from build123d import *

# Parameters (mm, degrees)
SKETCH2_R           = 15
SKETCH1_R           = 25
SKETCH3_R           = 15
BOSS_EXTRUDE1_DEPTH = 5
FILLET1_R           = 10
SKETCH4_R           = 1.75
CUT_EXTRUDE1_DEPTH  = 130
SKETCH5_R           = 4
CUT_EXTRUDE2_DEPTH  = 130
SKETCH6_R           = 22
BOSS_EXTRUDE2_DEPTH = 4
SKETCH7_R           = 17
BOSS_EXTRUDE3_DEPTH = 20
SKETCH15_W          = 8.431609766
SKETCH15_H          = 4
SKETCH15_W_2        = 8.578672696
SKETCH18_R          = 12.5
CUT_EXTRUDE5_DEPTH  = 20
SKETCH19_R          = 47.987160243
CUT_EXTRUDE6_DEPTH  = 44.301270362
SKETCH20_R          = 1.75
BOSS_EXTRUDE5_DEPTH = 4
CIRPATTERN3_COUNT   = 4
FILLET2_R           = 10
CHAMFER1_SIZE       = 0.5
SKETCH22_W          = 15
SKETCH22_H          = 8
BOSS_EXTRUDE6_DEPTH = 7.5
CHAMFER2_SIZE       = 3
CHAMFER3_SIZE       = 0.5
CUT_EXTRUDE8_START  = -0.1
SKETCH24_R          = 41.017326151
SKETCH24_R_2        = 17
CUT_EXTRUDE8_DEPTH  = 0.1
CHAMFER4_SIZE       = 0.5


with BuildPart() as part:
    # Sketch2 → Loft1 section 0
    with BuildSketch(Plane.XY.offset(20)):
        Circle(SKETCH2_R)
    # Sketch1 → Loft1 section 1
    with BuildSketch(Plane.XY):
        Circle(SKETCH1_R)
    loft()

    # Sketch3 → Boss-Extrude1 (add)
    with BuildSketch(Plane.XY.offset(20)):
        Circle(SKETCH3_R)
    extrude(amount=BOSS_EXTRUDE1_DEPTH)

    # Fillet1
    fillet1_edges = [part.edges().sort_by_distance(p)[0] for p in [
        (-15, 0, 20),
    ]]
    fillet(fillet1_edges, radius=FILLET1_R)

    # Sketch4 → Cut-Extrude1 (cut)
    with BuildSketch(Plane(origin=(0, 0, 0), x_dir=(-1, 0, 0), z_dir=(0, 0, -1))):
        with Locations((0, 20)):
            Circle(SKETCH4_R)
        with Locations((-20, 0)):
            Circle(SKETCH4_R)
        with Locations((0, -20)):
            Circle(SKETCH4_R)
        with Locations((20, 0)):
            Circle(SKETCH4_R)
    extrude(amount=-CUT_EXTRUDE1_DEPTH, mode=Mode.SUBTRACT)

    # Sketch5 → Cut-Extrude2 (cut)
    with BuildSketch(Plane(origin=(0, 0, 3), x_dir=(-1, 0, 0), z_dir=(0, 0, -1))):
        with Locations((0, 20)):
            Circle(SKETCH5_R)
        with Locations((20, 0)):
            Circle(SKETCH5_R)
        with Locations((-20, 0)):
            Circle(SKETCH5_R)
        with Locations((0, -20)):
            Circle(SKETCH5_R)
    extrude(amount=-CUT_EXTRUDE2_DEPTH, mode=Mode.SUBTRACT)

    # Sketch6 → Boss-Extrude2 (add)
    with BuildSketch(Plane.XY.offset(25)):
        Circle(SKETCH6_R)
    extrude(amount=BOSS_EXTRUDE2_DEPTH)

    # Sketch7 → Boss-Extrude3 (add)
    with BuildSketch(Plane.XY.offset(29)):
        Circle(SKETCH7_R)
    extrude(amount=BOSS_EXTRUDE3_DEPTH)

    # Sketch15 → Cut-Revolve1 (revolve, cut)
    with BuildSketch(Plane(origin=(0, 0, 0), x_dir=(1, 0, 0), z_dir=(0, 1, 0))):
        with Locations((-17.215804883, -35)):
            Rectangle(SKETCH15_W, SKETCH15_H)
        with Locations((-17.289336348, -43)):
            Rectangle(SKETCH15_W_2, SKETCH15_H)
    revolve(axis=Axis((0, 0, 29), (0, 0, 1)), mode=Mode.SUBTRACT)

    # Sketch18 → Cut-Extrude5 (cut)
    with BuildSketch(Plane(origin=(0, 0, 0), x_dir=(-1, 0, 0), z_dir=(0, 0, -1))):
        Circle(SKETCH18_R)
    extrude(amount=-CUT_EXTRUDE5_DEPTH, mode=Mode.SUBTRACT)

    # Sketch19 → Cut-Extrude6 (cut, through all)
    with BuildSketch(Plane(origin=(0, 0, 25), x_dir=(-1, 0, 0), z_dir=(0, 0, -1))):
        Circle(SKETCH19_R)
    extrude(amount=CUT_EXTRUDE6_DEPTH, mode=Mode.SUBTRACT)

    # Sketch20 → Boss-Extrude5 (add)
    with BuildSketch(Plane(origin=(0, 0, 25), x_dir=(-1, 0, 0), z_dir=(0, 0, -1))):
        with BuildLine():
            Line((-4, 30), (-4, 21.633307653))
            ThreePointArc((-4, 21.633307653), (0, 22), (4, 21.633307653))
            Line((4, 21.633307653), (4, 30))
            ThreePointArc((4, 30), (0, 34), (-4, 30))
        make_face()
        with Locations((0, 30)):
            Circle(SKETCH20_R, mode=Mode.SUBTRACT)
    boss_extrude5 = extrude(amount=-BOSS_EXTRUDE5_DEPTH)

    # CirPattern3: Boss-Extrude5 ×4 about axis
    cirpattern3_axis = Axis((0, 0, 0), (0, 0, 1))
    for i in range(1, CIRPATTERN3_COUNT):
        add(boss_extrude5.rotate(cirpattern3_axis, i * 360 / CIRPATTERN3_COUNT))

    # Fillet2
    fillet2_edges = [part.edges().sort_by_distance(p)[0] for p in [
        (-4, 21.633307653, 27),
        (4, 21.633307653, 27),
        (-21.633307653, -4, 27),
        (-21.633307653, 4, 27),
        (4, -21.633307653, 27),
        (-4, -21.633307653, 27),
        (21.633307653, 4, 27),
        (21.633307653, -4, 27),
    ]]
    fillet(fillet2_edges, radius=FILLET2_R)

    # Chamfer1
    chamfer1_edges = [part.edges().sort_by_distance(p)[0] for p in [
        (-17, 0, 49),
        (-17, 0, 37),
        (-17, 0, 33),
        (-17, 0, 45),
        (-17, 0, 41),
    ]]
    chamfer(chamfer1_edges, length=CHAMFER1_SIZE)

    # Sketch22 → Boss-Extrude6 (add, symmetric)
    with BuildSketch(Plane(origin=(0, 0, 0), x_dir=(1, 0, 0), z_dir=(0, 1, 0))):
        with Locations((0, -53)):
            Rectangle(SKETCH22_W, SKETCH22_H)
    extrude(amount=BOSS_EXTRUDE6_DEPTH, both=True)

    # Chamfer2
    chamfer2_edges = [part.edges().sort_by_distance(p)[0] for p in [
        (7.5, -7.5, 53),
        (-7.5, -7.5, 53),
        (7.5, 7.5, 53),
        (-7.5, 7.5, 53),
    ]]
    chamfer(chamfer2_edges, length=CHAMFER2_SIZE)

    # Chamfer3
    chamfer3_edges = [part.edges().sort_by_distance(p)[0] for p in [
        (7.5, 0, 49),
        (7.5, 0, 57),
        (0, -7.5, 57),
        (0, -7.5, 49),
        (0, 7.5, 57),
        (-7.5, 0, 57),
        (-6, 6, 57),
        (-6, -6, 57),
        (6, 6, 57),
        (6, -6, 57),
        (0, 7.5, 49),
        (-7.5, 0, 49),
        (6, -6, 49),
        (6, 6, 49),
        (-6, -6, 49),
        (-6, 6, 49),
    ]]
    chamfer(chamfer3_edges, length=CHAMFER3_SIZE)

    # Sketch24 → Cut-Extrude8 (cut)
    with BuildSketch(Plane.XY.offset(29).offset(CUT_EXTRUDE8_START)):
        Circle(SKETCH24_R)
        with Locations(Location((0, 0, 0), (0, 0, 180))):
            Circle(SKETCH24_R_2, mode=Mode.SUBTRACT)
    extrude(amount=CUT_EXTRUDE8_DEPTH, mode=Mode.SUBTRACT)

    # Chamfer4
    chamfer4_edges = [part.edges().sort_by_distance(p)[0] for p in [
        (0, 34, 25),
        (4, 29.38749457, 25),
        (1.75, 30, 25),
        (-34, 0, 25),
        (-29.38749457, 4, 25),
        (-30, 1.75, 25),
        (0, -34, 25),
        (-4, -29.38749457, 25),
        (-1.75, -30, 25),
        (34, 0, 25),
        (29.38749457, -4, 25),
        (30, -1.75, 25),
        (15.556349186, 15.556349186, 25),
        (29.38749457, 4, 25),
        (15.556349186, -15.556349186, 25),
        (4, -29.38749457, 25),
        (-15.556349186, -15.556349186, 25),
        (-29.38749457, -4, 25),
        (-15.556349186, 15.556349186, 25),
        (-4, 29.38749457, 25),
        (23.471688281, 5.522087521, 25),
        (23.471688281, -5.522087521, 25),
        (5.522087521, -23.471688281, 25),
        (-5.522087521, -23.471688281, 25),
        (-23.471688281, -5.522087521, 25),
        (-23.471688281, 5.522087521, 25),
        (-5.522087521, 23.471688281, 25),
        (5.522087521, 23.471688281, 25),
    ]]
    chamfer(chamfer4_edges, length=CHAMFER4_SIZE)


solid = part.part
Geometry: final body of the model. Coordinates: model frame, mm. A direction names the side the tool comes from. Give positions to 0.01 mm unless a question says otherwise; leave off trailing zeros. Loops run counter-clockwise (first coordinate to the right, second up) from the corner with the lowest first, then second, coordinate; pieces in that order, holes last. Notation, with made-up numbers: M 60,49.5 L 119,49.5 A7 ccw 119,56.5 Z; hole C 27.5,-31.5 d6. An arc over 180 degrees is marked long. Put each result on its own line as item: value. Start each with the question number.
1) Cut plane A-A (x = 0). Give the number of separate pieces and of enclosed holes in the cut face, then the cut area to 3 significant figures.
2) Contact query for flat-ended pins moving along their axis: pin 1 (2 mm diameter, centred on x = 0, z = 53, fed in from +Y); pin 2 (1.3 mm diameter, centred on x = 29, z = 27, fed in from +Y); pin 3 (7.5 mm diameter, centred on y = -2, z = 53.5, fed in from +X); pin 4 (3 mm diameter, centred on x = -19.5, z = 33.5, fed in from -Y). Output: stop coordinate, or through.
3) Cut plane C-C (z = 34.5). Output: boundary loops of the cut face in (x, y).
4) Pull-direction query (X, two-part tool) for faces 1 (the cylindrical face through (10.316, 7.91, 34.972)), 2 (the flat face through (0.1, 13.4, 33)), 3 (the cylindrical face through (-1.29, -31.18, 27.18)); classes: pulls with the +X half, pulls with the -X half, needs draft (parallel to the pull), parting line crosses it, or undercut.
5) Ray query, line 1 along Z through (x, y) = (1, 15); line 2 along Y through (x, z) = (0, 26.2); line 3 along Y through (x, z) = (-30, 27). Return the intervals inside material, ascending.
6) Access query for faces 4 (the cylindrical face through (-15.48, 15.63, 27.18)), 5 (the cylindrical face through (9.139, 14.334, 46.979)), 6 (the flat face through (7.5, 0, 53)). Directions: +Z, -Z, +X, -X, +Y, -Y. A direction counts if a zero-diameter tool reaches every point of the face in a straight line with its end or side. Return the directions, or none.
Verdict:
1. separate pieces: 3
1. enclosed holes: 0
1. area: 975 mm2
2. pin 1: y = 7.5
2. pin 2: y = 4.01
2. pin 3: x = 7.5
2. pin 4: through
3. outline: C 0,0 d26
4. face 1: parting line crosses it
4. face 2: needs draft
4. face 3: undercut
5. line 1: 25 to 33, 37 to 41, 45 to 49
5. line 2: -34 to -31.75, -28.25 to 28.25, 31.75 to 34
5. line 3: -4 to -1.75, 1.75 to 4
6. face 4: +Z, -Z, -X, +Y
6. face 5: +Z
6. face 6: +Z, +X, +Y, -Y
